Input: part model. Units: mm. Frame: model coordinates. Face numbers are marked on the shaded views. Give positions to 0.01 mm unless a question says otherwise; leave off trailing zeros. Loops run counter-clockwise (first coordinate to the right, second up) from the corner with the lowest first, then second, coordinate; pieces in that order, holes last. Notation, with made-up numbers: M 74.5,-38.5 L 116.5,-38.5 A14 ccw 116.5,-14.5 Z; hole C 42.25,13 d8. An arc over 180 degrees is marked long. Answer as a JSON object with one key per item and string values. Group by question number.
1) Section query B-B on y = 105. Count the separate pieces of the cut face and the enclosed holes in it, plus the area to 3 significant figures.
2) Section query C-C on y = 59.5. Return loops of the section in (x, z), plus the area to 3 significant figures.
3) Section query D-D on x = 100. Return loops of the section in (y, z), plus the area to 3 significant figures.
4) Draft query along Y for the marked faces 1 and 2. Return one class per face: +Y half, -Y half, draft (parallel to the pull), parting line (faces both ways), or undercut.
5) First-contact query: P1, Ø1.5, axis at x = 133, z = -4, coming from the +Y side; P2, Ø1.5, axis at x = 100, z = -4, coming from the -Y side; P3, Ø1, axis at y = 101, z = -7, coming from the -X side; P4, Ø12, axis at x = 158.5, y = 95.5, coming from the -Z side. Flat tips, straight axial feed; report the tip coordinate or a pass-through.
6) Ray query, L1, parallel to Y at x = 55, z = -1.5; L2, parallel to Y at x = 91, z = -4; L3, parallel to X at y = 47, z = -5.5. Return the intervals inside material, ascending.
Autodesk Fusion 360 part; units mm, degrees
sketch "Sketch1" plane through (0, 0, 0) normal (0, 0, 1) x (1, 0, 0)
  line L0 (4.6495, 21.5388) -> (192.9573, 21.5388)
  line L1 (197.9573, 26.5388) -> (197.9573, 115.0177)
  line L2 (192.9573, 120.0177) -> (4.6495, 120.0177)
  line L3 (-0.3505, 115.0177) -> (-0.3505, 26.5388)
  line L4 (10, 110) -> (38, 110)
  line L5 (38, 110) -> (38, 85)
  line L6 (38, 85) -> (10, 85)
  line L7 (10, 85) -> (10, 110)
  circle A0 centre (55, 105) radius 2.5
  circle A1 centre (55, 90) radius 3.0001
  circle A2 centre (100, 105) radius 2.5
  circle A3 centre (100, 49) radius 2.5
  circle A4 centre (155, 105) radius 2.5
  circle A5 centre (155, 49) radius 2.5
  arc A6 (4.6495, 120.0177) -> (-0.3505, 115.0177) centre (4.6495, 115.0177) ccw
  arc A7 (197.9573, 115.0177) -> (192.9573, 120.0177) centre (192.9573, 115.0177) ccw
  arc A8 (192.9573, 21.5388) -> (197.9573, 26.5388) centre (192.9573, 26.5388) ccw
  arc A9 (-0.3505, 26.5388) -> (4.6495, 21.5388) centre (4.6495, 26.5388) ccw
  line L8 (4.6495, 115.0177) -> (192.9573, 115.0177)
  line L9 (192.9573, 115.0177) -> (192.9573, 26.5388)
  line L10 (192.9573, 26.5388) -> (4.6495, 26.5388)
  line L11 (4.6495, 26.5388) -> (4.6495, 115.0177)
  line L12 (8, 112) -> (189.9275, 112)
  line L13 (189.9275, 112) -> (189.9275, 29.9593)
  line L14 (189.9275, 29.9593) -> (8, 29.9593)
  line L15 (8, 29.9593) -> (8, 112)
  circle A10 centre (20, 40) radius 2
  circle A11 centre (20, 40) radius 3
  circle A12 centre (20, 75) radius 2
  circle A13 centre (20, 75) radius 3
  circle A14 centre (55, 40) radius 2
  circle A15 centre (55, 40) radius 3
  circle A16 centre (55, 75) radius 2
  circle A17 centre (55, 75) radius 3
  dimension "d1" = 5
  dimension "d2" = 6.0002
  dimension "d3" = 5
  dimension "d4" = 5
  dimension "d5" = 5
  dimension "d6" = 5
  dimension "d7" = 5
extrude "Extrude8" add sketch "Sketch1" against normal blind 3 contours L0 L1 L2 L3 A6 A7 A8 A9 | L12 L13 L14 L15 makes body 1 at (67.4187, 23.2054, 0) makes body 2 at (118.9226, 85.7441, 0)
extrude "Extrude9" add sketch "Sketch1" against normal blind 6 contours L8 L9 L10 L11 bodies 1 2
extrude "Extrude10" add sketch "Sketch1" against normal blind 5 contours A11 | A13 | A15 | A17 bodies 1
extrude "Extrude11" add sketch "Sketch1" against normal blind 8 contours A10 | A12 | A14 | A16 bodies 1
extrude "Extrude12" add sketch "Sketch1" against normal blind 8 contours A2 | A3 | A4 | A5 bodies 1
chamfer "Chamfer4" distance 2 angle 45 1 edges at (10, 97.5, -3) on bodies 1
chamfer "Chamfer5" distance 2 angle 45 1 edges at (23, 110, -3) on bodies 1
chamfer "Chamfer6" distance 2 angle 45 1 edges at (38, 98.5, -3) on bodies 1
chamfer "Chamfer7" distance 2 angle 45 1 edges at (24, 85, -3) on bodies 1
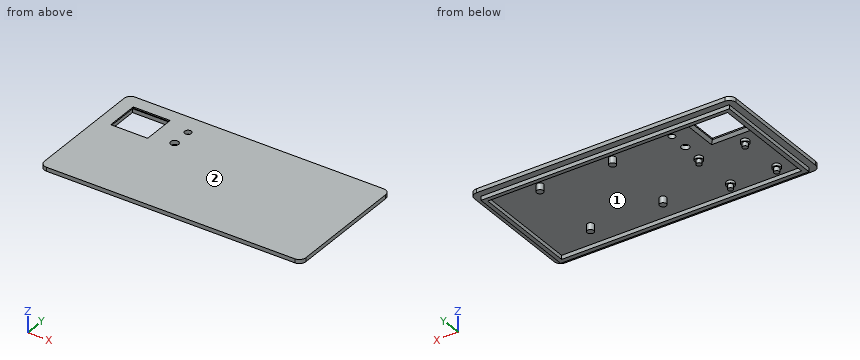
Output:
{
 "1": {"separate pieces": "3", "enclosed holes": "0", "area": "561 mm^2"},
 "2": {"outline": "M -0.35,-3 L 4.65,-3 L 4.65,-6 L 8,-6 L 8,-3 L 189.93,-3 L 189.93,-6 L 192.96,-6 L 192.96,-3 L 197.96,-3 L 197.96,0 L -0.35,0 Z", "area": "614 mm^2"},
 "3": {"outline": "M 21.54,-3 L 26.54,-3 L 26.54,-6 L 29.96,-6 L 29.96,-3 L 46.5,-3 L 46.5,-8 L 51.5,-8 L 51.5,-3 L 102.5,-3 L 102.5,-8 L 107.5,-8 L 107.5,-3 L 112,-3 L 112,-6 L 115.02,-6 L 115.02,-3 L 120.02,-3 L 120.02,0 L 21.54,0 Z", "area": "365 mm^2"},
 "4": {"face 1": "undercut", "face 2": "draft"},
 "5": {"P1": "stops at y = 115.02", "P2": "stops at y = 26.54", "P3": "passes through", "P4": "stops at z = -3"},
 "6": {"L1": "y = 21.54 to 87, 93 to 102.5, 107.5 to 120.02", "L2": "y = 26.54 to 29.96, 112 to 115.02", "L3": "x = 4.65 to 8, 98.5 to 101.5, 153.5 to 156.5, 189.93 to 192.96"}
}
